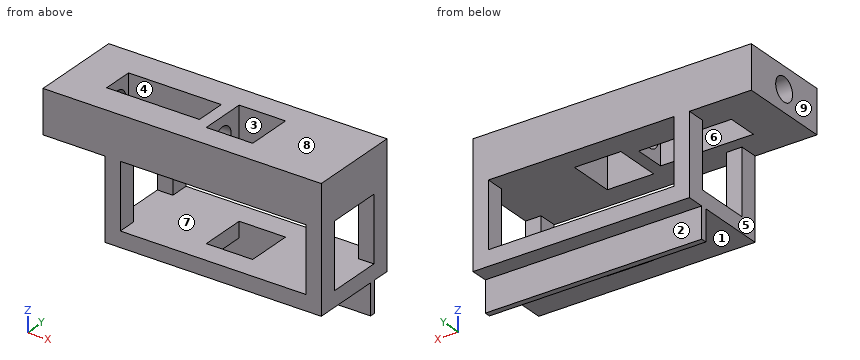
from build123d import *

# Parameters (mm, degrees)
SKETCH1_W                = 88.9
SKETCH1_H                = 38.1
SKETCH1_W_2              = 25.4
BOSS_EXTRUDE1_DEPTH      = 17.78
SKETCH2_W                = 38.1
SKETCH2_H                = 12.7
SKETCH2_W_2              = 6.35
SKETCH2_H_2              = 7.62
SKETCH2_W_3              = 19.05
SKETCH2_H_3              = 19.05
CUT_EXTRUDE1_DEPTH       = 41.402
SKETCH3_W                = 19.05
SKETCH3_H                = 19.05
BOSS_EXTRUDE2_DEPTH      = 6.35
SPRINGPLUNGER_HOLE_REACH = 132.755
SKETCH6_R                = 4.8895
SKETCH8_W                = 6.35
SKETCH8_H                = 7.62
SUPPORT_DEPTH            = 50.8
SKETCH10_W               = 88.9
SKETCH10_H               = 2.413
BOSS_EXTRUDE3_DEPTH      = 12.7


with BuildPart() as part:
    # Sketch1 → Boss-Extrude1 (new body)
    with BuildSketch(Plane.XY):
        with Locations((44.45, 19.05)):
            Rectangle(SKETCH1_W, SKETCH1_H)
        with Locations((-12.7, 19.05)):
            Rectangle(SKETCH1_W_2, SKETCH1_H)
    extrude(amount=-BOSS_EXTRUDE1_DEPTH)

    # Sketch2 → Cut-Extrude1 (cut)
    with BuildSketch(Plane.XY):
        with Locations((10.795, 19.05)):
            Rectangle(SKETCH2_W, SKETCH2_H)
        with Locations((3.175, 34.29)):
            Rectangle(SKETCH2_W_2, SKETCH2_H_2)
        with Locations((3.175, 3.81)):
            Rectangle(SKETCH2_W_2, SKETCH2_H_2)
        with Locations((44.45, 19.05)):
            Rectangle(SKETCH2_W_3, SKETCH2_H_3)
        with Locations((85.725, 34.29)):
            Rectangle(SKETCH2_W_2, SKETCH2_H_2)
        with Locations((85.725, 3.81)):
            Rectangle(SKETCH2_W_2, SKETCH2_H_2)
    extrude(amount=-CUT_EXTRUDE1_DEPTH, mode=Mode.SUBTRACT)

    # SpringPlunger Hole: up to this face of the body (flat: up to its plane)
    springplunger_hole_end = Plane(part.part.faces().sort_by_distance((34.925, 19.05, -8.89))[0])
    # Sketch6 → SpringPlunger Hole (cut, up to the picked face)
    with BuildSketch(Plane.ZY.offset(25.4), mode=Mode.PRIVATE) as springplunger_hole_sk1:
        with Locations((-8.89, 19.05)):
            Circle(SKETCH6_R)
    springplunger_hole_tool1 = split(extrude(springplunger_hole_sk1.sketch, amount=-SPRINGPLUNGER_HOLE_REACH, mode=Mode.PRIVATE), bisect_by=springplunger_hole_end, keep=Keep.BOTH, mode=Mode.PRIVATE)
    add(springplunger_hole_tool1.solids().sort_by(Axis((-25.4, 19.05, -8.89), (1, 0, 0)))[0], mode=Mode.SUBTRACT)



with BuildPart() as body_2:
    # Sketch3 → Boss-Extrude2 (new body)
    with BuildSketch(Plane.XY.offset(-50.8)):
        Polygon((0, 30.48), (0, 7.62), (6.35, 7.62), (6.35, 0), (82.55, 0), (82.55, 7.62), (88.9, 7.62), (88.9, 30.48), (82.55, 30.48), (82.55, 38.1), (6.35, 38.1), (6.35, 30.48), align=None)
        with Locations((44.45, 19.05)):
            Rectangle(SKETCH3_W, SKETCH3_H, mode=Mode.SUBTRACT)
    extrude(amount=BOSS_EXTRUDE2_DEPTH)


with BuildPart() as part_1:
    add(part.part)

    add(body_2.part)  # Support merges body 2
    # Sketch8 → Support (add)
    with BuildSketch(Plane.XY):
        with Locations((3.175, 34.29)):
            Rectangle(SKETCH8_W, SKETCH8_H)
        with Locations((85.725, 34.29)):
            Rectangle(SKETCH8_W, SKETCH8_H)
        with Locations((85.725, 3.81)):
            Rectangle(SKETCH8_W, SKETCH8_H)
        with Locations((3.175, 3.81)):
            Rectangle(SKETCH8_W, SKETCH8_H)
    extrude(amount=-SUPPORT_DEPTH)

    # Sketch10 → Boss-Extrude3 (add)
    with BuildSketch(Plane(origin=(0, 0, -50.8), x_dir=(-1, 0, 0), z_dir=(0, 0, -1))):
        with Locations((-44.45, 29.7815)):
            Rectangle(SKETCH10_W, SKETCH10_H)
    extrude(amount=BOSS_EXTRUDE3_DEPTH)


solid = part_1.part
The listing builds one solid part. Answer for the finished solid, in the listing's coordinates (mm). Face numbers are marked on the shaded views. A direction names the side the tool comes from. Coordinates: 2 decimals unless noted, no trailing zeros. Loops run counter-clockwise (first coordinate to the right, second up) from the corner with the lowest first, then second, coordinate; pieces in that order, holes last.
1) Determine the mould class of the marked faces 6, 7, 8 and 9 for opening direction X: pulls with the +X half, pulls with the -X half, needs draft (parallel to the pull), parting line crosses it, or undercut.
2) Find section C-C on z = -22. Write down the section's boundary in (x, y), then the cut area to 3 significant figures.
3) Find section A-A on x = 37. Write down the section's boundary in (y, z) (3 decimals).
4) Find section B-B on x = 10.5. Write down the section's boundary in (y, z) (3 decimals), then the cut area to 3 significant figures.
5) Find section D-D on y = 19.05. Give the number of separate pieces and of enclosed holes in the cut face, then the cut area to 3 significant figures.
6) A tool of negligible diameter and unlimited length cuts with its end or side. For the marked faces 1, 2, 3, 4 and 5, from which of +Z, -Z, +X, -X, +Y, -Y can it reach the whole face along a straight path? Write none if from no direction.
7) Flat-ended cylindrical pins translate along their axes: pin 1 Ø2 at (x, y) = (27, 35) entering from -Z; pin 2 Ø3 at (y, z) = (23.5, -47.5) entering from -X; pin 3 Ø6 at (y, z) = (19.05, -8.89) entering from -X (3 decimals). Find the tip coordinate at first contact, or state that the pin passes through.
8) Find the intervals of material crossed by L1, parallel to X at y = 13, z = -9 (3 decimals); L2, parallel to Z at x = 31, y = 19; L3, parallel to Y at x = -13.5, z = -8.89, in increasing order.
Values:
1. face 6: undercut
1. face 7: undercut
1. face 8: needs draft
1. face 9: pulls with the -X half
2. outline: (0, 0) - (6.35, 0) - (6.35, 7.62) - (0, 7.62) - close; (0, 30.48) - (6.35, 30.48) - (6.35, 38.1) - (0, 38.1) - close; (82.55, 0) - (88.9, 0) - (88.9, 7.62) - (82.55, 7.62) - close; (82.55, 30.48) - (88.9, 30.48) - (88.9, 38.1) - (82.55, 38.1) - close
2. area: 194 mm2
3. outline: (0, -50.8) - (9.525, -50.8) - (9.525, -44.45) - (0, -44.45) - close; (0, -17.78) - (9.525, -17.78) - (9.525, 0) - (0, 0) - close; (28.575, -63.5) - (30.988, -63.5) - (30.988, -50.8) - (38.1, -50.8) - (38.1, -44.45) - (28.575, -44.45) - close; (28.575, -17.78) - (38.1, -17.78) - (38.1, 0) - (28.575, 0) - close
4. outline: (0, -50.8) - (28.575, -50.8) - (28.575, -63.5) - (30.988, -63.5) - (30.988, -50.8) - (38.1, -50.8) - (38.1, -44.45) - (0, -44.45) - close; (0, -17.78) - (12.7, -17.78) - (12.7, 0) - (0, 0) - close; (25.4, -17.78) - (38.1, -17.78) - (38.1, 0) - (25.4, 0) - close
4. area: 724 mm2
5. separate pieces: 7
5. enclosed holes: 0
5. area: 1,240 mm2
6. face 1: -Z, +X, -X, -Y
6. face 2: -Z, +X, -X, +Y
6. face 3: +Z, -Z
6. face 4: +Z
6. face 5: -Z, -X, +Y, -Y
7. pin 1: stops at z = -50.8
7. pin 2: stops at x = 0
7. pin 3: stops at x = 53.975
8. L1: x = -25.4 to -8.255, 29.845 to 34.925, 53.975 to 88.9
8. L2: z = -50.8 to -44.45, -17.78 to -13.78, -4 to 0
8. L3: y = 0 to 14.16, 23.94 to 38.1
